Input: part model. Units: mm. Frame: model coordinates. A direction names the side the tool comes from. Coordinates: 2 decimals unless noted, no trailing zeros. Loops run counter-clockwise (first coordinate to the right, second up) from the corner with the lowest first, then second, coordinate; pieces in that order, holes last.
Autodesk Inventor part; units mm, degrees
ref_plane "Start Plane" through (0, 0, 0) normal (1, 0, 0) x (0, 1, 0)
ref_plane "XZ Plane" through (0, 0, 0) normal (0, 1, 0) x (-1, 0, 0)
ref_plane "XY Plane" through (0, 0, 0) normal (0, 0, 1) x (1, 0, 0)
sketch "Main Sketch" plane through (0, 0, 0) normal (0, 0, 1) x (1, 0, 0)
  line L0 (0, 0) -> (79, 0)
  line L1 (0, 0) -> (0, 6.5)
  line L2 (0, 6.5) -> (10, 6.5)
  line L3 (10, 6.5) -> (10, 7.8)
  line L4 (56, 7.8) -> (56, 7.5)
  line L5 (10, 7.8) -> (56, 7.8)
  line L6 (69, 7.5) -> (69, 6.5)
  line L7 (56, 7.5) -> (69, 7.5)
  line L8 (79, 6.5) -> (79, 0)
  line L9 (69, 6.5) -> (79, 6.5)
  dimension "d3" = 13
  dimension "d4" = 15.6
  dimension "d5" = 15
  dimension "d6" = 13
revolve "Revolution1" add sketch "Main Sketch" angle 360 about axis through (0, 0, 0) along (1, 0, 0)
chamfer "Chamfer4" distance 0.5 angle 45 1 edges at (0, -6.5, 0) measured on face at (3.3333, 6.4158, -1.0427)
chamfer "Chamfer2" distance 0.5 angle 45 1 edges at (10, -6.5, 0) measured on face at (3.6667, 6.4789, -0.523)
chamfer "Chamfer3" distance 0.5 angle 45 1 edges at (10, -7.8, 0) measured on face at (25.3333, 7.699, -1.2512)
properties part number "Pedales - Eje" material "Steel"
Item 1: Section query A-A (z = 0). Output: boundary loops of the cut face in (x, y), then the cut area to 3 significant figures.
Result:
outline: (0, -6) - (0.5, -6.5) - (9.5, -6.5) - (10, -7) - (10, -7.3) - (10.5, -7.8) - (56, -7.8) - (56, -7.5) - (69, -7.5) - (69, -6.5) - (79, -6.5) - (79, 6.5) - (69, 6.5) - (69, 7.5) - (56, 7.5) - (56, 7.8) - (10.5, 7.8) - (10, 7.3) - (10, 7) - (9.5, 6.5) - (0.5, 6.5) - (0, 6) - close
area: 1,170 mm2
Item 2: Line query: L1, parallel to Y at x = 75, z = -2.5; L2, parallel to Y at x = 41.5, z = 0.5; L3, parallel to Z at x = 43.5, y = -5. Output: solid intervals per line, ascending.
Result:
L1: y = -6 to 6
L2: y = -7.78 to 7.78
L3: z = -5.99 to 5.99
Item 3: Contact query for flat-ended pins moving along their axis: P1, Ø1, axis at x = 31.5, z = 4, coming from the -Y side; P2, Ø1, axis at x = 15, y = 5, coming from the -Z side; P3, Ø2, axis at x = 24, y = 2.5, coming from the -Z side. Output: stop coordinate, or through.
Result:
P1: stops at y = -6.97
P2: stops at z = -6.37
P3: stops at z = -7.65
Item 4: Section query D-D (x = 39). Output: boundary loops of the cut face in (y, z), then the cut area to 3 significant figures.
Result:
outline: circle Ø15.6 at (0, 0)
area: 191 mm2
Item 5: Reachability of faces 1 (the face through (62.591, -7.493, 0.33)), 2 (the face through (79, 0, 0)), 3 (the face through (5.063, -5.158, -3.955)) from +Z, -Z, +X, -X, +Y, -Y: full face, straight path, thin tool, end or side. Return the list, or none.
Result:
face 1: +X
face 2: +Z, -Z, +X, +Y, -Y
face 3: -X
Item 6: Section query C-C (x = 66.5). Output: boundary loops of the cut face in (y, z), then the cut area to 3 significant figures.
Result:
outline: circle Ø15 at (0, 0)
area: 177 mm2
